Design review of the part built by this model. Coordinates are the model's own, in mm. A direction names the side the tool comes from. Coordinates: 2 decimals unless noted, no trailing zeros. Order: outer loops, then holes, each group sorted by start corner. A loop starts at its lowest first (then second) coordinate and runs counter-clockwise, first axis right, second up. Notation, with made-up numbers: M 1.25,70 L 40.25,70 A22 ccw 40.25,86 Z; hole C 27.5,-12.5 d8. An arc over 180 degrees is marked long. Use CSV: the item, a comma, the result in double quotes.
Autodesk Inventor part; units mm, degrees
ref_plane "YZ Plane" through (0, 0, 0) normal (1, 0, 0) x (0, 1, 0)
ref_plane "XZ Plane" through (0, 0, 0) normal (0, 1, 0) x (-1, 0, 0)
ref_plane "XY Plane" through (0, 0, 0) normal (0, 0, 1) x (1, 0, 0)
sketch "Sketch1" plane through (0, 0, 0) normal (0, 0, 1) x (1, 0, 0)
  line L0 (-21.15, -21.15) -> (21.15, -21.15)
  line L1 (21.15, -21.15) -> (21.15, 21.15)
  line L2 (21.15, 21.15) -> (-21.15, 21.15)
  line L3 (-21.15, 21.15) -> (-21.15, -21.15)
  line L4 (-21.15, -21.15) -> (21.15, 21.15) construction
  line L5 (21.15, -21.15) -> (-21.15, 21.15) construction
  point P0 (0, 0)
  dimension "d0" = 42.3
  dimension "d1" = 42.3
extrude "Extrusion1" add sketch "Sketch1" along normal blind 40
chamfer "Chamfer1" distance 5 angle 45 4 edges at (21.15, -21.15, 20) (-21.15, -21.15, 20) (21.15, 21.15, 20) (-21.15, 21.15, 20)
sketch "Sketch2" plane through (0, 0, 40) normal (0, 0, 1) x (1, 0, 0)
  circle A0 centre (0, 0) radius 18
  dimension "d7" = 36
extrude "Extrusion2" add sketch "Sketch2" along normal blind 35
sketch "Sketch3" plane through (0, 0, 40) normal (0, 0, 1) x (1, 0, 0)
  circle A0 centre (0, 0) radius 18
  line L0 (-21.15, 16.15) -> (-16.15, 21.15)
  line L1 (-21.15, 16.15) -> (-21.15, -16.15)
  line L2 (-16.15, -21.15) -> (-21.15, -16.15)
  line L3 (-16.15, -21.15) -> (16.15, -21.15)
  line L4 (21.15, -16.15) -> (16.15, -21.15)
  line L5 (21.15, -16.15) -> (21.15, 16.15)
  line L6 (16.15, 21.15) -> (21.15, 16.15)
  line L7 (16.15, 21.15) -> (-16.15, 21.15)
  line L8 (-15.7358, 20.15) -> (-20.15, 15.7358)
  line L9 (-20.15, 15.7358) -> (-20.15, -15.7358)
  line L10 (-20.15, -15.7358) -> (-15.7358, -20.15)
  line L11 (-15.7358, -20.15) -> (15.7358, -20.15)
  line L12 (15.7358, -20.15) -> (20.15, -15.7358)
  line L13 (20.15, -15.7358) -> (20.15, 15.7358)
  line L14 (20.15, 15.7358) -> (15.7358, 20.15)
  line L15 (15.7358, 20.15) -> (-15.7358, 20.15)
  dimension "d10" = 1
extrude "Extrusion3" add sketch "Sketch3" along normal blind 5 contours L15 L14 L13 L12 L11 L10 L9 L8
sketch "Sketch4" plane through (0, 0, 45) normal (0, 0, 1) x (1, 0, 0)
  line L0 (-15.5, -15.5) -> (15.5, -15.5) construction
  line L1 (15.5, -15.5) -> (15.5, 15.5) construction
  line L2 (15.5, 15.5) -> (-15.5, 15.5) construction
  line L3 (-15.5, 15.5) -> (-15.5, -15.5) construction
  line L4 (-15.5, -15.5) -> (15.5, 15.5) construction
  line L5 (15.5, -15.5) -> (-15.5, 15.5) construction
  point P0 (0, 0)
  dimension "d13" = 31
  dimension "d14" = 31
hole "Hole1" at (-15.5, 15.5, 45) at (15.5, 15.5, 45) at (-15.5, -15.5, 45) at (15.5, -15.5, 45) direction (0, 0, -1) diameter 5 depth 0.5
sketch "Sketch5" plane through (0, 0, 75) normal (0, 0, 1) x (1, 0, 0)
  circle A0 centre (0, 0) radius 11
  dimension "d22" = 22
extrude "Extrusion4" add sketch "Sketch5" along normal blind 2
sketch "Sketch6" plane through (0, 0, 77) normal (0, 0, 1) x (1, 0, 0)
  circle A0 centre (0, 0) radius 4
  dimension "d25" = 8
extrude "Extrusion5" add sketch "Sketch6" along normal blind 18
sketch "Sketch7" plane through (0, 0, 95) normal (0, 0, 1) x (1, 0, 0)
  line L0 (-2.6458, 4) -> (2.6458, 4)
  line L1 (2.6458, 4) -> (2.6458, 3)
  line L2 (2.6458, 3) -> (-2.6458, 3)
  line L3 (-2.6458, 3) -> (-2.6458, 4)
  circle A0 centre (0, 0) radius 4
  line L4 (0, 0) -> (0, 4)
  circle A1 centre (0, 0) radius 4
  point P0 (0, 3)
  dimension "d28" = 7
extrude "Extrusion6" cut sketch "Sketch7" against normal blind 15 contours L0 A0 L3 | L0 L1 A0 | L4 L2 A0 | A0 L2 L4
chamfer "Chamfer2" distance 0.5 angle 45 2 edges at (3.6458, 1.6458, 95) (-1.6458, -3.6458, 95)
chamfer "Chamfer3" distance 1 angle 45 8 edges at (0, 21.15, 0) (18.65, 18.65, 0) (21.15, 0, 0) (-21.15, 0, 0) (-18.65, 18.65, 0) (18.65, -18.65, 0) (0, -21.15, 0) (-18.65, -18.65, 0)
scale "Scale1" factors (25.4, 25.4, 25.4) then translate (0, 0, -1464) bodies 1
properties part number "motor con reductora"
(1) Add section A-A on y = 0. State the section outline as (x, z) points, and give its area (3 significant figures).
The answers:
outline,"M -537.21,-1438.6 L -511.81,-1464 L 511.81,-1464 L 537.21,-1438.6 L 537.21,-448 L 511.81,-448 L 511.81,-321 L 457.2,-321 L 457.2,441 L 279.4,441 L 279.4,491.8 L 101.6,491.8 L 101.6,936.3 L 88.9,949 L -88.9,949 L -101.6,936.3 L -101.6,491.8 L -279.4,491.8 L -279.4,441 L -457.2,441 L -457.2,-321 L -511.81,-321 L -511.81,-448 L -537.21,-448 Z"
area,"2,040,000 mm2"
(2) For faces 1 (the face through (-511.81, 6, -385)), 2 (the face through (-455, 456.5, -385.4)), 3 (the face through (-221.722, 170.011, 466.044)), 4 (the face through (1, 76.2, 761)), 5 (the face through (511.81, -6, -385)), list the 3-axis set-ups (+Z, -Z, +X, -X, +Y, -Y) from which the entire face can be reached by the end or side of a thin tool; tool diameter is ignored.
The answers:
face 1,"+Z, -X, +Y, -Y"
face 2,"+Z, -X, +Y"
face 3,"+Z"
face 4,"+Z, +X, -X, +Y"
face 5,"+Z, +X, +Y, -Y"
(3) Add section D-D on y = 365. State the section outline as (x, z) points, and give its area (3 significant figures).
The answers:
outline,"M -537.21,-1438.6 L -511.81,-1464 L 511.81,-1464 L 537.21,-1438.6 L 537.21,-448 L 511.81,-448 L 511.81,-321 L 450.34,-321 L 450.34,-333.7 L 337.06,-333.7 L 337.06,-321 L 275.33,-321 L 275.33,441 L -275.33,441 L -275.33,-321 L -337.06,-321 L -337.06,-333.7 L -450.34,-333.7 L -450.34,-321 L -511.81,-321 L -511.81,-448 L -537.21,-448 Z"
area,"1,640,000 mm2"
(4) Add section B-B on z = -892.5. State the section outline as (x, y) points, and give its area (3 significant figures).
The answers:
outline,"M -537.21,-410.21 L -410.21,-537.21 L 410.21,-537.21 L 537.21,-410.21 L 537.21,410.21 L 410.21,537.21 L -410.21,537.21 L -537.21,410.21 Z"
area,"1,120,000 mm2"
(5) Clearance check with flat-ended pins moving along their axes: P1, Ø6, axis at x = 318, z = -396, coming from the +Y side; P2, Ø2, axis at x = 73.5, y = -191, coming from the +Z side; P3, Ø5, axis at y = -376.5, z = -176, coming from the -X side (3 decimals). State where each tip first meets the part, or that it passes through.
The answers:
P1,"stops at y = 511.81"
P2,"stops at z = 491.8"
P3,"stops at x = -262.975"
(6) Add section C-C on x = -133. State the section outline as (y, z) points.
The answers:
outline,"M -537.21,-1438.6 L -511.81,-1464 L 511.81,-1464 L 537.21,-1438.6 L 537.21,-448 L 511.81,-448 L 511.81,-321 L 437.43,-321 L 437.43,441 L 245.71,441 L 245.71,491.8 L -245.71,491.8 L -245.71,441 L -437.43,441 L -437.43,-321 L -511.81,-321 L -511.81,-448 L -537.21,-448 Z"
(7) Wall thickness on probe 1 along Y at (x, z) = (393, -327); probe 2 along Y at (x, z) = (49, 520): over which ranges is each line inside the solid? List them lowest first.
The answers:
probe 1,"y = -511.81 to -457.2, -330.2 to 330.2, 457.2 to 511.81"
probe 2,"y = -89 to 89"
(8) The part is to be moulded in two halves that separate along Y. For faces 6 (the face through (-412.77, -454.27, -327.44)), 7 (the face through (-520, 3, -448)), 8 (the face through (456.5, 455, -385.4)), say which applies: pulls with the +Y half, pulls with the -Y half, needs draft (parallel to the pull), parting line crosses it, or undercut.
The answers:
face 6,"undercut"
face 7,"needs draft"
face 8,"pulls with the +Y half"
